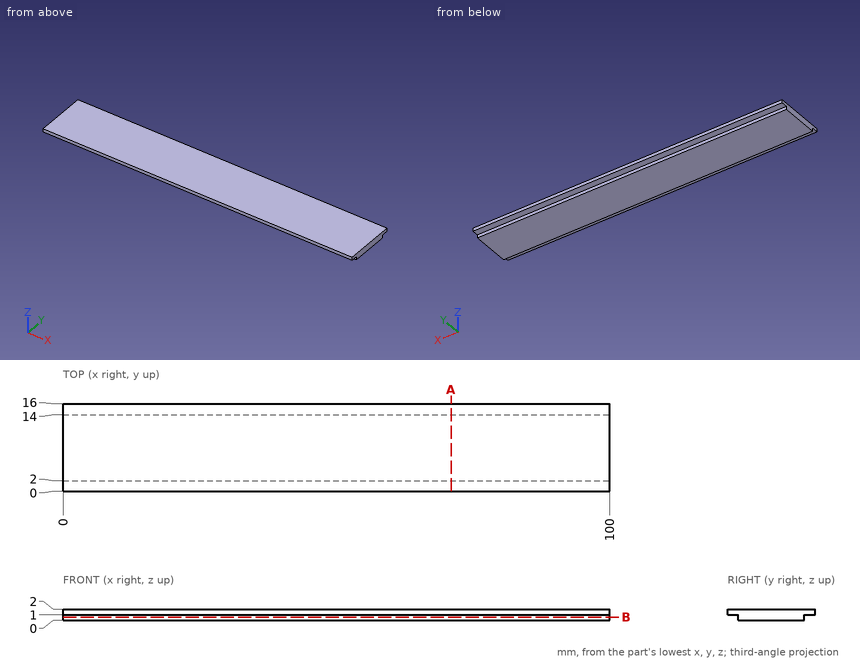
Answer from the drawing. Dimensions are ordinates in mm from the lowest x, y and z of the part. Round coordinates to 2 decimals unless told otherwise and drop trailing zeros. Order: outer loops, then holes, each group sorted by start corner. A loop starts at its lowest first (then second) coordinate and runs counter-clockwise, first axis right, second up. Notation, with made-up numbers: (-24, -20) - (18, -20) arc R18 ccw to (18, -9) - close; hole circle Ø5 at (20, 69). An arc over 180 degrees is marked (long way). Put each result on its own line as item: value. Start each with the question number.
(1) Given P1, Ø1.6, axis at x = 27, y = 0.5, coming from the -Z side; P2, Ø1, axis at x = 78.5, z = 1, coming from the -Y side, each flat-ended and moving along its own axis, determine where each tip first touches the part or whether it passes through.
(2) Find section A-A (x = 71). Give the vertices of the cut face in (y, z), plus the area to 3 significant figures.
(3) Find section B-B (z = 0.6). Give the vertices of the cut face in (x, y).
(4) A straight line is drawn through the part: probe 1 along Y at (x, z) = (92.5, 0.7). Find the intervals that lie inside material, in ascending order. Write a range as from..to.
Reply:
1. P1: z = 1
1. P2: y = 0
2. outline: (0, 1) - (2, 1) - (2, 0) - (14, 0) - (14, 1) - (16, 1) - (16, 2) - (0, 2) - close
2. area: 28.0 mm^2
3. outline: (0, 2) - (100, 2) - (100, 14) - (0, 14) - close
4. probe 1: 2..14
